Read the model definition and answer for the solid it produces. Units are mm, in the model's axes. A direction names the side the tool comes from. Round coordinates to 2 decimals unless told otherwise and drop trailing zeros. Order: outer loops, then holes, each group sorted by start corner. A loop starts at its lowest first (then second) coordinate and runs counter-clockwise, first axis right, second up. Notation, with made-up numbers: (20.25, 19) -> (76.25, 19) arc R18 cw to (76.25, 51) -> close; hole circle Ø7 at (39.25, 69.5). An arc over 180 degrees is marked (long way). One line per item, written item: value. Start each with the question number.
1. The mould has two halves that part along X. Classify faces 3 (the face through (1.25, 2.38, 2.13)), 4 (the face through (4, 7, 2)), 5 (the face through (-0.867, 15.534, 3.905)), 6 (the face through (-1.32, 1.26, -2.24)): released by +X, released by -X, zero draft, split by the parting line, or undercut.
2. Flat-ended cylindrical pins translate along their axes: pin 1 Ø5 at (x, y) = (4, 11) entering from +Z; pin 2 Ø3 at (x, y) = (4, 12.5) entering from +Z. Find the tip coordinate at first contact, or state that the pin passes through.
3. Section C-C (y = 23.5) is taken. Give the vertices of the cut face in (x, z).
4. Consider line 1 (Y direction, x = -4.25, z = 1.5); line 2 (Z direction, x = 5, y = 4.75); line 3 (X direction, y = 1.25, z = 1). Determine where each line is inside the solid, lowest interval first.
5. Section B-B (y = 2.75) is taken. Give the vertices of the cut face in (x, z).
6. Section A-A (z = 0) is taken. Give the vertices of the cut face in (x, y).
7. For faces 1 (the face through (1.802, 3.458, 5.723)), 2 (the face through (0, 2.5, 0)), determine the directions among +Z, -Z, +X, -X, +Y, -Y from which every point of the face is accessible in a straight line to the end or side of a thin tool.
from build123d import *

# Parameters (mm, degrees)
SKETCH1_R               = 6
BOSS_EXTRUDE1_DEPTH     = 25
CHAMFER1_SIZE           = 0.5
CUT_EXTRUDE1_DEPTH      = 27.400757565
CUT_EXTRUDE1_DEPTH_BACK = 2.5
CHAMFER2_SIZE           = 0.25


# Read off the part's stored shape, not the designer's step: M8x1.25 Machine Threads Stud2
with BuildPart() as part:
    # Sketch1 → Boss-Extrude1 (new body)
    with BuildSketch(Plane(origin=(0, 0, 0), x_dir=(1, 0, 0), z_dir=(0, 1, 0))):
        with Locations(Location((0, 0, 0), (0, 0, 270))):
            Circle(SKETCH1_R)
    extrude(amount=BOSS_EXTRUDE1_DEPTH)

    # M8x1.25 Machine Threads Stud2 outline → M8x1.25 Machine Threads Stud2 (revolve, cut)
    with BuildSketch(Plane.XY):
        Polygon((6, 25), (3.3095, 25), (4, 24.3095), (4, 7), (6, 7), align=None)
    revolve(axis=Axis((0, 0, 0), (0, 1, 0)), mode=Mode.SUBTRACT)

    # Chamfer1
    chamfer1_edges = [part.edges().sort_by_distance(p)[0] for p in [
        (0, 0, -6),
        (0, 7, -6),
    ]]
    chamfer(chamfer1_edges, length=CHAMFER1_SIZE)

    # Sketch6 → Cut-Extrude1 (cut, two sides: drawn at the far end of the back side and taken through both)
    with BuildSketch(Plane.XZ.offset(-CUT_EXTRUDE1_DEPTH_BACK)):
        Polygon((0, -3), (2.598076211, -1.5), (2.598076211, 1.5), (0, 3), (-2.598076211, 1.5), (-2.598076211, -1.5), align=None)
    extrude(amount=CUT_EXTRUDE1_DEPTH + CUT_EXTRUDE1_DEPTH_BACK, mode=Mode.SUBTRACT)

    # Chamfer2
    chamfer2_edges = [part.edges().sort_by_distance(p)[0] for p in [
        (-2.598076211, 0, 0),
        (-1.299038106, 0, 2.25),
        (1.299038106, 0, 2.25),
        (2.598076211, 0, 0),
        (1.299038106, 0, -2.25),
        (-1.299038106, 0, -2.25),
        (-1.299038106, 2.5, -2.25),
        (1.299038106, 2.5, -2.25),
        (2.598076211, 2.5, 0),
        (1.299038106, 2.5, 2.25),
        (-1.299038106, 2.5, 2.25),
        (-2.598076211, 2.5, 0),
    ]]
    chamfer(chamfer2_edges, length=CHAMFER2_SIZE)


solid = part.part
Answer:
1. face 3: undercut
1. face 4: zero draft
1. face 5: split by the parting line
1. face 6: undercut
2. pin 1: z = 3.71
2. pin 2: z = 3.12
3. outline: circle Ø8 at (0, 0)
4. line 1: 0 to 7
4. line 2: -3.32 to 3.32
4. line 3: -5.92 to -2.6, 2.6 to 5.92
5. outline: circle Ø12 at (0, 0)
6. outline: (-6, 0.5) -> (-5.5, 0) -> (-2.85, 0) -> (-2.6, 0.25) -> (-2.6, 2.25) -> (-2.35, 2.5) -> (2.35, 2.5) -> (2.6, 2.25) -> (2.6, 0.25) -> (2.85, 0) -> (5.5, 0) -> (6, 0.5) -> (6, 6.5) -> (5.5, 7) -> (4, 7) -> (4, 24.31) -> (3.31, 25) -> (-3.31, 25) -> (-4, 24.31) -> (-4, 7) -> (-5.5, 7) -> (-6, 6.5) -> close
7. face 1: +Y, -Y
7. face 2: -Y
